Here's how the part is built. I have some questions about the finished solid (model axes, mm). Coordinates: 2 decimals unless noted, no trailing zeros. Loops run counter-clockwise (first coordinate to the right, second up) from the corner with the lowest first, then second, coordinate; pieces in that order, holes last.
from build123d import *

# Parameters (mm, degrees)
SKETCH1_W           = 12
SKETCH1_H           = 3
BOSS_EXTRUDE1_DEPTH = 3
FILLET1_RADIUS      = 1.5
FILLET1_LENGTH      = 3
FILLET2_RADIUS      = 1.5
FILLET2_LENGTH      = 3
CHAMFER2_SIZE       = 0.2


with BuildPart() as part:
    # Sketch1 → Boss-Extrude1 (new body)
    with BuildSketch(Plane(origin=(0, 0, 0), x_dir=(1, 0, 0), z_dir=(0, 1, 0))):
        Rectangle(SKETCH1_W, SKETCH1_H)
    extrude(amount=BOSS_EXTRUDE1_DEPTH)

    # Fillet1: full round fillet: the end face becomes a half cylinder, R = half its width
    fillet1_face = Plane((-6, 1.5, 0), x_dir=(0, -1, 0), z_dir=(-1, 0, 0))  # on the end face: x along it, z out of the body
    fillet1_slab = fillet1_face.offset(-FILLET1_RADIUS / 2) * Box(FILLET1_LENGTH, 2 * FILLET1_RADIUS, FILLET1_RADIUS, mode=Mode.PRIVATE)  # the body's end, R deep
    fillet1_round = Plane((-4.5, 1.5, 0), x_dir=(-1, 0, 0), z_dir=(0, -1, 0)) * Cylinder(FILLET1_RADIUS, FILLET1_LENGTH, mode=Mode.PRIVATE)  # its axis R under the face
    add(fillet1_slab - fillet1_round, mode=Mode.SUBTRACT)

    # Fillet2: full round fillet: the end face becomes a half cylinder, R = half its width
    fillet2_face = Plane((6, 1.5, 0), x_dir=(0, 1, 0), z_dir=(1, 0, 0))  # on the end face: x along it, z out of the body
    fillet2_slab = fillet2_face.offset(-FILLET2_RADIUS / 2) * Box(FILLET2_LENGTH, 2 * FILLET2_RADIUS, FILLET2_RADIUS, mode=Mode.PRIVATE)  # the body's end, R deep
    fillet2_round = Plane((4.5, 1.5, 0), x_dir=(1, 0, 0), z_dir=(0, 1, 0)) * Cylinder(FILLET2_RADIUS, FILLET2_LENGTH, mode=Mode.PRIVATE)  # its axis R under the face
    add(fillet2_slab - fillet2_round, mode=Mode.SUBTRACT)

    # Chamfer2
    chamfer2_edges = [part.edges().sort_by_distance(p)[0] for p in [
        (0, 0, 1.5),
        (0, 3, 1.5),
        (-6, 3, 0),
        (-6, 0, 0),
        (0, 0, -1.5),
        (0, 3, -1.5),
        (6, 0, 0),
        (6, 3, 0),
    ]]
    chamfer(chamfer2_edges, length=CHAMFER2_SIZE)


solid = part.part
Q1. Please list where these lines run through material, in increasing order: probe 1 along X at (y, z) = (2.55, -0.1); probe 2 along Z at (x, y) = (-5.25, 2.7); probe 3 along X at (y, z) = (0.7, -0.7).
Q2. Suppose I cut it at A-A on y = 2.55. Write out the boundary of the cut face in (x, z), and give its area (3 significant figures).
Q3. Will this pin go through, and if not, where does the flat tip stop? P1, Ø1, axis at y = 0.5, z = 1, coming from the -X side.
Check values:
1. probe 1: x = -6 to 6
1. probe 2: z = -1.3 to 1.3
1. probe 3: x = -5.83 to 5.83
2. outline: (-4.5, -1.5) - (4.5, -1.5) arc R1.5 ccw to (4.5, 1.5) - (-4.5, 1.5) arc R1.5 ccw to start
2. area: 34.1 mm2
3. P1: stops at x = -5.91
